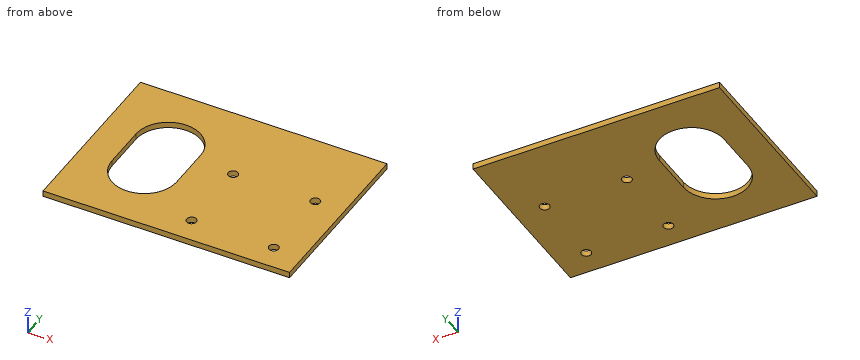
from build123d import *

# Parameters (mm, degrees)
SKETCH1_W           = 84
SKETCH1_H           = 61
SKETCH1_R           = 1.65
BOSS_EXTRUDE1_DEPTH = 2


with BuildPart() as part:
    # Sketch1 → Boss-Extrude1 (new body)
    with BuildSketch(Plane.XY):
        with Locations((-110.4, 45.7)):
            Rectangle(SKETCH1_W, SKETCH1_H)
        with Locations((-106.4, 23.7)):
            Circle(SKETCH1_R, mode=Mode.SUBTRACT)
        with Locations((-78.4, 23.7)):
            Circle(SKETCH1_R, mode=Mode.SUBTRACT)
        with Locations((-78.4, 49.7)):
            Circle(SKETCH1_R, mode=Mode.SUBTRACT)
        with Locations((-106.4, 49.7)):
            Circle(SKETCH1_R, mode=Mode.SUBTRACT)
        with BuildLine():
            Line((-119.4, 53.2), (-119.4, 38.2))
            ThreePointArc((-119.4, 38.2), (-130.4, 27.2), (-141.4, 38.2))
            Line((-141.4, 38.2), (-141.4, 53.2))
            ThreePointArc((-141.4, 53.2), (-130.4, 64.2), (-119.4, 53.2))
        make_face(mode=Mode.SUBTRACT)
    extrude(amount=BOSS_EXTRUDE1_DEPTH)


solid = part.part
Read the model definition and answer for the solid it produces. Units are mm, in the model's axes. Round coordinates to 2 decimals unless told otherwise and drop trailing zeros. Write each loop counter-clockwise with the first axis right and the second up, starting at its lowest first coordinate (ties: lowest second). Pieces come first, ordered by that corner, then holes.
1. The part is cut by section D-D, the plane y = 49.7. Determine the outline of the cut face in (x, z).
2. The part is cut by section A-A, the plane x = -78.4. Determine the outline of the cut face in (y, z).
3. Straight lines are drawn through the part: L1, parallel to Y at x = -78.4, z = 0.6; L2, parallel to X at y = 30.5, z = 0.7; L3, parallel to Y at x = -138, z = 0.8. For each, find the intervals that lie inside material, in ascending order.
4. The part is cut by section C-C, the plane z = 0.75. Determine the outline of the cut face in (x, y).
5. The part is cut by section B-B, the plane y = 23.7. Determine the outline of the cut face in (x, z).
Values:
1. outline: (-152.4, 0) - (-141.4, 0) - (-141.4, 2) - (-152.4, 2) - close; (-119.4, 0) - (-108.05, 0) - (-108.05, 2) - (-119.4, 2) - close; (-104.75, 0) - (-80.05, 0) - (-80.05, 2) - (-104.75, 2) - close; (-76.75, 0) - (-68.4, 0) - (-68.4, 2) - (-76.75, 2) - close
2. outline: (15.2, 0) - (22.05, 0) - (22.05, 2) - (15.2, 2) - close; (25.35, 0) - (48.05, 0) - (48.05, 2) - (25.35, 2) - close; (51.35, 0) - (76.2, 0) - (76.2, 2) - (51.35, 2) - close
3. L1: y = 15.2 to 22.05, 25.35 to 48.05, 51.35 to 76.2
3. L2: x = -152.4 to -138.26, -122.54 to -68.4
3. L3: y = 15.2 to 30.25, 61.15 to 76.2
4. outline: (-152.4, 15.2) - (-68.4, 15.2) - (-68.4, 76.2) - (-152.4, 76.2) - close; hole (-141.4, 38.2) arc R11 ccw to (-119.4, 38.2) - (-119.4, 53.2) arc R11 ccw to (-141.4, 53.2) - close; hole circle Ø3.3 at (-106.4, 23.7); hole circle Ø3.3 at (-106.4, 49.7); hole circle Ø3.3 at (-78.4, 23.7); hole circle Ø3.3 at (-78.4, 49.7)
5. outline: (-152.4, 0) - (-108.05, 0) - (-108.05, 2) - (-152.4, 2) - close; (-104.75, 0) - (-80.05, 0) - (-80.05, 2) - (-104.75, 2) - close; (-76.75, 0) - (-68.4, 0) - (-68.4, 2) - (-76.75, 2) - close
